The listing builds one solid part. Answer for the finished solid, in the listing's coordinates (mm). Coordinates: 2 decimals unless noted, no trailing zeros. Order: outer loops, then holes, each group sorted by start corner. A loop starts at its lowest first (then second) coordinate and runs counter-clockwise, first axis right, second up.
from build123d import *

# Parameters (mm, degrees)
SKETCH_1_R      = 11.05
SKETCH_1_R_2    = 1.65
SKETCH_1_R_3    = 4.05
SKETCH_1_R_4    = 2.65
EXTRUDE_1_DEPTH = 6


with BuildPart() as part:
    # 草图1 → 凸台-拉伸1 (new body)
    with BuildSketch(Plane(origin=(0, 0, 0), x_dir=(1, 0, 0), z_dir=(0, 1, 0))):
        with BuildLine():
            Line((-35, -42), (35, -42))
            ThreePointArc((35, -42), (38.535533906, -40.535533906), (40, -37))
            Line((40, -37), (40, 20))
            ThreePointArc((40, 20), (38.535533906, 23.535533906), (35, 25))
            Line((35, 25), (-35, 25))
            ThreePointArc((-35, 25), (-38.535533906, 23.535533906), (-40, 20))
            Line((-40, 20), (-40, -37))
            ThreePointArc((-40, -37), (-38.535533906, -40.535533906), (-35, -42))
        make_face()
        with Locations(Location((0, 0, 0), (0, 0, 270))):
            Circle(SKETCH_1_R, mode=Mode.SUBTRACT)
        with Locations(Location((-15.5, 15.5, 0), (0, 0, 270))):
            Circle(SKETCH_1_R_2, mode=Mode.SUBTRACT)
        with Locations(Location((15.5, 15.5, 0), (0, 0, 270))):
            Circle(SKETCH_1_R_2, mode=Mode.SUBTRACT)
        with Locations(Location((15.5, -15.5, 0), (0, 0, 270))):
            Circle(SKETCH_1_R_2, mode=Mode.SUBTRACT)
        with Locations(Location((-15.5, -15.5, 0), (0, 0, 270))):
            Circle(SKETCH_1_R_2, mode=Mode.SUBTRACT)
        with Locations(Location((-25, 0, 0), (0, 0, 270))):
            Circle(SKETCH_1_R_3, mode=Mode.SUBTRACT)
        with Locations(Location((-25, 16, 0), (0, 0, 270))):
            Circle(SKETCH_1_R_4, mode=Mode.SUBTRACT)
        with Locations(Location((-25, -16, 0), (0, 0, 90))):
            Circle(SKETCH_1_R_4, mode=Mode.SUBTRACT)
        with Locations(Location((25, 0, 0), (0, 0, 90))):
            Circle(SKETCH_1_R_3, mode=Mode.SUBTRACT)
        with Locations(Location((25, -16, 0), (0, 0, 270))):
            Circle(SKETCH_1_R_4, mode=Mode.SUBTRACT)
        with Locations(Location((25, 16, 0), (0, 0, 90))):
            Circle(SKETCH_1_R_4, mode=Mode.SUBTRACT)
        with Locations(Location((-35, 19, 0), (0, 0, 270))):
            Circle(SKETCH_1_R_2, mode=Mode.SUBTRACT)
        with Locations(Location((-35, -36, 0), (0, 0, 270))):
            Circle(SKETCH_1_R_2, mode=Mode.SUBTRACT)
        with Locations(Location((35, -36, 0), (0, 0, 90))):
            Circle(SKETCH_1_R_2, mode=Mode.SUBTRACT)
        with Locations(Location((35, 19, 0), (0, 0, 90))):
            Circle(SKETCH_1_R_2, mode=Mode.SUBTRACT)
        with Locations(Location((-10, -32, 0), (0, 0, 270))):
            Circle(SKETCH_1_R_4, mode=Mode.SUBTRACT)
        with Locations(Location((-30, -32, 0), (0, 0, 270))):
            Circle(SKETCH_1_R_4, mode=Mode.SUBTRACT)
        with Locations(Location((30, -32, 0), (0, 0, 90))):
            Circle(SKETCH_1_R_4, mode=Mode.SUBTRACT)
        with Locations(Location((10, -32, 0), (0, 0, 90))):
            Circle(SKETCH_1_R_4, mode=Mode.SUBTRACT)
    extrude(amount=EXTRUDE_1_DEPTH)


solid = part.part
(1) Find the intervals of material crossed by probe 1 along X at (y, z) = (2.6, 32); probe 2 along Z at (x, y) = (35, 1.6); probe 3 along X at (y, z) = (3.95, -15.5), in increasing order.
(2) Find section B-B on z = 32. Determine the outline of the cut face in (x, y), then the cut area to 3 significant figures.
(3) The mould has two halves that part along X. Classify faces 1 (the cylindrical face through (38, 3, 41)), 2 (the cylindrical face through (-39, 3, 40)), 3 (the cylindrical face through (-10.787, 2.958, -2.395)), 4 (the flat face through (-1, 0, 15)): pulls with the +X half, pulls with the -X half, needs draft (parallel to the pull), parting line crosses it, or undercut.
(4) Given pin 1 Ø3 at (x, z) = (10, 32) entering from +Y; pin 2 Ø8.5 at (x, z) = (25, -16) entering from +Y, each flat-ended and moving along its own axis, determine where each tip first touches the part or whether it passes through.
(5) Find section D-D on z = -15.5. Determine the outline of the cut face in (x, y), then the cut area to 3 significant figures.
(6) Find section C-C on y = 1.4. Count the separate pieces of the cut face and the enclosed holes in it, then the cut area to 3 significant figures.
(7) Find section A-A on x = 25. Determine the outline of the cut face in (y, z), then the cut area to 3 significant figures.
Resolved:
1. probe 1: x = -40 to -32.65, -27.35 to -12.65, -7.35 to 7.35, 12.65 to 27.35, 32.65 to 40
1. probe 2: z = -25 to -20.65, -17.35 to 34.35, 37.65 to 42
1. probe 3: x = -40 to -27.6, -22.4 to -17.15, -13.85 to 13.85, 17.15 to 22.4, 27.6 to 40
2. outline: (-40, 0) - (-32.65, 0) - (-32.65, 6) - (-40, 6) - close; (-27.35, 0) - (-12.65, 0) - (-12.65, 6) - (-27.35, 6) - close; (-7.35, 0) - (7.35, 0) - (7.35, 6) - (-7.35, 6) - close; (12.65, 0) - (27.35, 0) - (27.35, 6) - (12.65, 6) - close; (32.65, 0) - (40, 0) - (40, 6) - (32.65, 6) - close
2. area: 353 mm2
3. face 1: pulls with the +X half
3. face 2: pulls with the -X half
3. face 3: undercut
3. face 4: needs draft
4. pin 1: passes through
4. pin 2: stops at y = 6
5. outline: (-40, 0) - (-27.6, 0) - (-27.6, 6) - (-40, 6) - close; (-22.4, 0) - (-17.15, 0) - (-17.15, 6) - (-22.4, 6) - close; (-13.85, 0) - (13.85, 0) - (13.85, 6) - (-13.85, 6) - close; (17.15, 0) - (22.4, 0) - (22.4, 6) - (17.15, 6) - close; (27.6, 0) - (40, 0) - (40, 6) - (27.6, 6) - close
5. area: 378 mm2
6. separate pieces: 1
6. enclosed holes: 19
6. area: 4,610 mm2
7. outline: (0, -25) - (6, -25) - (6, -18.65) - (0, -18.65) - close; (0, -13.35) - (6, -13.35) - (6, -4.05) - (0, -4.05) - close; (0, 4.05) - (6, 4.05) - (6, 13.35) - (0, 13.35) - close; (0, 18.65) - (6, 18.65) - (6, 42) - (0, 42) - close
7. area: 290 mm2
